```python
from build123d import *

# Parameters (mm, degrees)
BOSS_EXTRUDE1_DEPTH = 2.5
CUT_EXTRUDE1_DEPTH  = 2.5


with BuildPart() as part:
    # Sketch1 → Boss-Extrude1 (new body)
    with BuildSketch(Plane.XY):
        Polygon((-60, -100), (-20, -100), (-20, -97.5), (-2.1, -97.5), (-2.1, -92.5), (-4, -92.5), (-4, -87.5), (-2.1, -87.5), (-2.1, -77.5), (0, -77.5), (2.1, -77.5), (2.1, -87.5), (4, -87.5), (4, -92.5), (2.1, -92.5), (2.1, -97.5), (20, -97.5), (20, -100), (60, -100), (60, -97.5), (100, -97.5), (100, 100), (-100, 100), (-100, -97.5), (-60, -97.5), align=None)
    extrude(amount=BOSS_EXTRUDE1_DEPTH)

    # Sketch4 → Cut-Extrude1 (cut)
    with BuildSketch(Plane(origin=(0, 0, 0), x_dir=(-1, 0, 0), z_dir=(0, 0, -1))):
        Polygon((-80, 0), (-100, 0), (-100, -2.1), (-95, -2.1), (-95, -4), (-90, -4), (-90, -2.1), (-80, -2.1), align=None)
        Polygon((-95, 2.1), (-100, 2.1), (-100, 0), (-80, 0), (-80, 2.1), (-90, 2.1), (-90, 4), (-95, 4), align=None)
        Polygon((-95, 62.1), (-100, 62.1), (-100, 57.9), (-95, 57.9), (-95, 56), (-90, 56), (-90, 57.9), (-80, 57.9), (-80, 62.1), (-90, 62.1), (-90, 64), (-95, 64), align=None)
        Polygon((-95, -57.9), (-100, -57.9), (-100, -62.1), (-95, -62.1), (-95, -64), (-90, -64), (-90, -62.1), (-80, -62.1), (-80, -57.9), (-90, -57.9), (-90, -56), (-95, -56), align=None)
        Polygon((95, 57.9), (100, 57.9), (100, 62.1), (95, 62.1), (95, 64), (90, 64), (90, 62.1), (80, 62.1), (80, 57.9), (90, 57.9), (90, 56), (95, 56), align=None)
        Polygon((95, -2.1), (100, -2.1), (100, 2.1), (95, 2.1), (95, 4), (90, 4), (90, 2.1), (80, 2.1), (80, -2.1), (90, -2.1), (90, -4), (95, -4), align=None)
        Polygon((100, -62.1), (100, -57.9), (95, -57.9), (95, -56), (90, -56), (90, -57.9), (80, -57.9), (80, -62.1), (90, -62.1), (90, -64), (95, -64), (95, -62.1), align=None)
    extrude(amount=-CUT_EXTRUDE1_DEPTH, mode=Mode.SUBTRACT)


solid = part.part
```
Build history of the part. All positions in model axes, mm. Give positions to 0.01 mm unless a question says otherwise; leave off trailing zeros. Loops run counter-clockwise (first coordinate to the right, second up) from the corner with the lowest first, then second, coordinate; pieces in that order, holes last. Notation, with made-up numbers: (10, -38) -> (62, -38) arc R21 ccw to (62, -22) -> close; hole circle Ø3 at (33, 79). An arc over 180 degrees is marked (long way). One line per question, with ' | ' between items. Start each with the question number.
1) Probe L1, parallel to Y at x = -90.5, z = 1.75; L2, parallel to Y at x = 89.5, z = 0.9; L3, parallel to X at y = -79, z = 0.4. List the from-to ranges inside material, lowest first.
2) Pin check, flat tips, straight feed: pin 1 (1 mm diameter, centred on x = 5.5, z = 0.5, fed in from -Y); pin 2 (1.2 mm diameter, centred on y = 59.5, z = 1.5, fed in from -X); pin 3 (1.2 mm diameter, centred on y = 0, z = 2, fed in from +X). Stop position of each tip, or through.
3) Cut at B-B (x = 86.5). Give the cut face in (y, z).
4) Cut at A-A (y = -84). Give the cut face in (x, z).
Return value:
1) L1: -97.5 to -64, -56 to -4, 4 to 56, 64 to 100 | L2: -97.5 to -62.1, -57.9 to -2.1, 2.1 to 57.9, 62.1 to 100 | L3: -100 to -2.1, 2.1 to 100
2) pin 1: y = -97.5 | pin 2: x = -80 | pin 3: x = 80
3) outline: (-97.5, 0) -> (-62.1, 0) -> (-62.1, 2.5) -> (-97.5, 2.5) -> close; (-57.9, 0) -> (-2.1, 0) -> (-2.1, 2.5) -> (-57.9, 2.5) -> close; (2.1, 0) -> (57.9, 0) -> (57.9, 2.5) -> (2.1, 2.5) -> close; (62.1, 0) -> (100, 0) -> (100, 2.5) -> (62.1, 2.5) -> close
4) outline: (-100, 0) -> (-2.1, 0) -> (-2.1, 2.5) -> (-100, 2.5) -> close; (2.1, 0) -> (100, 0) -> (100, 2.5) -> (2.1, 2.5) -> close
